Part model, mm, in its own coordinate system. A direction names the side the tool comes from. Coordinates: 2 decimals unless noted, no trailing zeros. Loops run counter-clockwise (first coordinate to the right, second up) from the corner with the lowest first, then second, coordinate; pieces in that order, holes last. Notation, with made-up numbers: M -20,48.5 L -13,48.5 A22 cw -13,64.5 Z; hole C 2,57.5 d9. An arc over 180 degrees is marked long. Answer as CSV lines item,"result". Start each with the question number.
from build123d import *

# Parameters (mm, degrees)
SUSP_FR_UCA_BALL_JOINT_PROFILE_R  = 17
SUSP_FR_LCA_BALL_JOINT_PROFILE_R  = 17
SUSP_FR_UPRIGHT_KINGPIN_START     = -189.376138003
SUSP_FR_UPRIGHT_KINGPIN_OUTLINE_R = 17
SUSP_FR_UPRIGHT_KINGPIN_DEPTH     = 234.300819272
SUSP_FR_UPRIGHT_SPINDLE_PROFILE_R = 20
SUSP_FR_UPRIGHT_ARM_PROFILE_R     = 9
SUSP_FR_HUB_PROFILE_R             = 55


# Read off the part's stored shape, not the designer's step: SUSP_FR_upright_kingpin
with BuildPart() as part:
    # SUSP_FR_UCA_ball_joint: sweep along a curve in space
    with BuildLine() as susp_fr_uca_ball_joint_path:
        Line((539.215175, -109.232527, -297.644798), (534.716988, -107.000649, -323.155287))
    # SUSP_FR_UCA_ball_joint profile (on start of the path) → SUSP_FR_UCA_ball_joint (sweep)
    with BuildSketch(Plane(origin=(539.215175, -109.232527, -297.644798), x_dir=(-0.9848077563247088, 0, 0.17364815888080395), z_dir=(-0.1730071904249639, 0.0858414606043016, -0.981172643168663))):
        Circle(SUSP_FR_UCA_BALL_JOINT_PROFILE_R)
    sweep(path=susp_fr_uca_ball_joint_path.line)


with BuildPart() as body_2:
    # SUSP_FR_LCA_ball_joint: sweep along a curve in space
    with BuildLine() as susp_fr_lca_ball_joint_path:
        Line((584.249094, -131.577136, -42.2447557), (579.750906, -129.345257, -67.7552443))
    # SUSP_FR_LCA_ball_joint profile (on start of the path) → SUSP_FR_LCA_ball_joint (sweep)
    with BuildSketch(Plane(origin=(584.249094, -131.577136, -42.2447557), x_dir=(-0.9848077492574088, 0, 0.17364819896145425), z_dir=(-0.17300722977562832, 0.08584149950700166, -0.9811726328265339))):
        Circle(SUSP_FR_LCA_BALL_JOINT_PROFILE_R)
    sweep(path=susp_fr_lca_ball_joint_path.line)


with BuildPart() as susp_fr_upright_kingpin_tool:
    # SUSP_FR_upright_kingpin outline → SUSP_FR_upright_kingpin (new body)
    with BuildSketch(Plane(origin=(0, 0, 0), x_dir=(0.9849205583589563, 0.01507857135321185, -0.17234886250807685), z_dir=(0.17300720713855208, -0.08584148118504255, 0.9811726384210254)).offset(SUSP_FR_UPRIGHT_KINGPIN_START)):
        with Locations((580.73578395, -134.758317541)):
            Circle(SUSP_FR_UPRIGHT_KINGPIN_OUTLINE_R)
    extrude(amount=SUSP_FR_UPRIGHT_KINGPIN_DEPTH)


with BuildPart() as part_1:
    add(part.part)


with BuildPart() as part_2:
    # SUSP_FR_upright_kingpin: joined with susp_fr_upright_kingpin_tool
    add(part_1.part.fuse(susp_fr_upright_kingpin_tool.part, body_2.part, tol=0.00001))

    # SUSP_FR_upright_spindle: sweep along a curve in space
    with BuildLine() as susp_fr_upright_spindle_path:
        Line((563.274706, -121.170213, -161.19642), (613.584449, -120.4, -170))
    # SUSP_FR_upright_spindle profile (on start of the path) → SUSP_FR_upright_spindle (sweep)
    with BuildSketch(Plane(origin=(563.274706, -121.170213, -161.19642), x_dir=(0.17236845779024892, 0, 0.9850325450252957), z_dir=(0.9849205586549441, 0.015078562779446367, -0.17234886156670431))):
        Circle(SUSP_FR_UPRIGHT_SPINDLE_PROFILE_R)
    sweep(path=susp_fr_upright_spindle_path.line)

    # SUSP_FR_upright_arm: sweep along a curve in space
    with BuildLine() as susp_fr_upright_arm_path:
        Line((575.079712, -127.027537, -94.2469055), (590.293517, -204.990503, -103.750386))
    # SUSP_FR_upright_arm profile (on start of the path) → SUSP_FR_upright_arm (sweep)
    with BuildSketch(Plane(origin=(575.079712, -127.027537, -94.2469055), x_dir=(-0.9814869975187847, -0.1915287803479187, 0), z_dir=(0.19017256143460165, -0.9745370695403799, -0.1187935055844866))):
        Circle(SUSP_FR_UPRIGHT_ARM_PROFILE_R)
    sweep(path=susp_fr_upright_arm_path.line)

    # SUSP_FR_hub: sweep along a curve in space
    with BuildLine() as susp_fr_hub_path:
        Line((593.591303, -120.4, -169.476461), (633.577596, -120.4, -170.523539))
    # SUSP_FR_hub profile (on start of the path) → SUSP_FR_hub (sweep)
    with BuildSketch(Plane(origin=(593.591303, -120.4, -169.476461), x_dir=(0.026176949998200826, 0, 0.9996573249312944), z_dir=(0.9996573249312944, 0, -0.026176949998200826))):
        Circle(SUSP_FR_HUB_PROFILE_R)
    sweep(path=susp_fr_hub_path.line)


solid = part_2.part
Q1. Tool access for faces 1 (the face through (613.6, -66.7, -181.9)), 2 (the face through (590.41, -204.95, -103.88)): list every direction of +Z, -Z, +X, -X, +Y, -Y with a clear straight run to the whole face (end or side of a thin tool).
Q2. Two-plate mould, pull along X, no slides. Class faces 3 (the face through (584.487, -131.34, -42.266)), 4 (the face through (576.801, -121.79, -183.848)), 5 (the face through (534.955, -106.764, -323.176)): +X half, -X half, draft (parallel to the pull), parting line (faces both ways), or undercut.
Q3. Flat gauge pins, fed straight in: P1, Ø5, axis at y = -138.5, z = -86.5, coming from the -X side; P2, Ø6, axis at y = -92.5, z = -212, coming from the -X side; P3, Ø8, axis at x = 540.5, z = -293.5, coming from the +Y side. Where does each tip first touch, or does it go through?
Q4. Wall check: L1, parallel to X at y = -103.5, z = -214; L2, parallel to Y at x = 604, z = -170.5; L3, parallel to X at y = -81, z = -142. Give the ranges that are in metal, low to high.
Q5. Slice it at A-A, the plane y = -77. Write the cut outline in (x, z), and give its area (3 significant figures).
Solved:
1,face 1,"none"
1,face 2,"-Z, +X, -Y"
2,face 3,"+X half"
2,face 4,"undercut"
2,face 5,"-X half"
3,P1,"stops at x = 561.46"
3,P2,"stops at x = 592.4"
3,P3,"stops at y = -92.2"
4,L1,"x = 542.64 to 564.89, 592.43 to 632.44"
4,L2,"y = -175.39 to -65.41"
4,L3,"x = 594.31 to 634.32"
5,outline,"M 592.71,-203.25 L 632.69,-204.3 L 634.46,-136.75 L 594.48,-135.7 Z"
5,area,"2,700 mm2"
